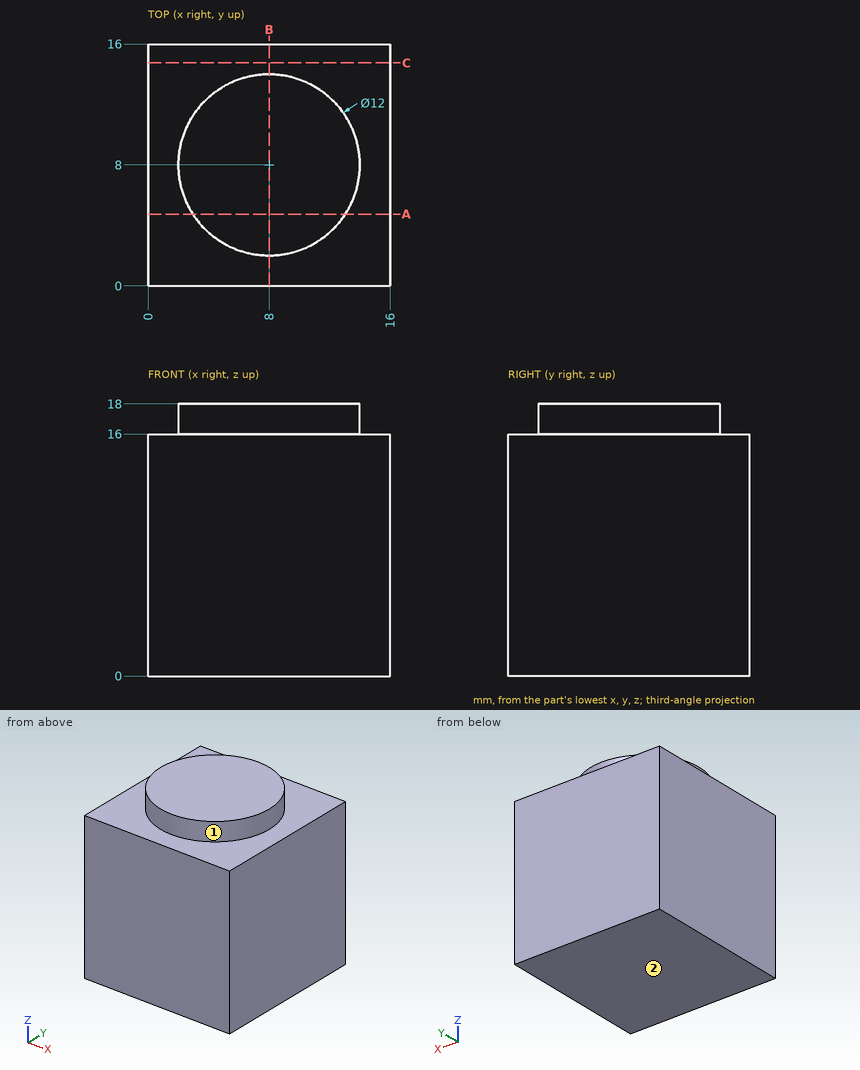
Can you work these out from the drawing? Everything is in mm from the part's minimum corner. A direction names the side the tool comes from. Round coordinates to 2 decimals unless told otherwise and drop trailing zeros. Loops run counter-clockwise (first coordinate to the right, second up) from the corner with the lowest first, then second, coordinate; pieces in that order, holes last. Notation, with made-up numbers: (22.25, 5) -> (26.25, 5) arc R20 cw to (26.25, 40) -> close; hole circle Ø1 at (53, 89.25). An arc over 180 degrees is marked (long way). Answer in a Markdown table with one row per item.
Item 1: On a 3-axis mill with a long thin cutter (end or side, diameter ignored), from which of +Z, -Z, +X, -X, +Y, -Y can I reach the whole of each face in a straight line? I mean the marked faces 1 and 2. Say none if no direction works.
Answer block:
| item | result |
|---|---|
| face 1 | +Z |
| face 2 | -Z, +X, -X, +Y, -Y |
Item 2: Suppose I cut it at C-C, the plane y = 14.75. List the corners of the cut face in (x, z) for me, plus the area to 3 significant figures.
Answer block:
| item | result |
|---|---|
| outline | (0, 0) -> (16, 0) -> (16, 16) -> (0, 16) -> close |
| area | 256 mm² |
Item 3: Will this pin go through, and if not, where does the flat tip stop? P1, Ø8, axis at y = 10.5, z = 13.5, coming from the -X side.
Answer block:
| item | result |
|---|---|
| P1 | x = 0 |
Item 4: If I drill on probe 1 along Z at (x, y) = (3.5, 14.25); probe 2 along X at (y, z) = (4.75, 16.75); probe 3 along X at (y, z) = (11.75, 16.75), over which ranges is the centre line in solid material (lowest first)?
Answer block:
| item | result |
|---|---|
| probe 1 | 0 to 16 |
| probe 2 | 2.96 to 13.04 |
| probe 3 | 3.32 to 12.68 |
Item 5: Suppose I cut it at B-B, the plane x = 8. List the corners of the cut face in (y, z) for me, plus the area to 3 significant figures.
Answer block:
| item | result |
|---|---|
| outline | (0, 0) -> (16, 0) -> (16, 16) -> (14, 16) -> (14, 18) -> (2, 18) -> (2, 16) -> (0, 16) -> close |
| area | 280 mm² |
Item 6: Suppose I cut it at A-A, the plane y = 4.75. List the corners of the cut face in (x, z) for me.
Answer block:
| item | result |
|---|---|
| outline | (0, 0) -> (16, 0) -> (16, 16) -> (13.04, 16) -> (13.04, 18) -> (2.96, 18) -> (2.96, 16) -> (0, 16) -> close |
